```python
from build123d import *

# Parameters (mm, degrees)
F1_DEPTH = 10
F2_R     = 25.98667
F3_DEPTH = 20


with BuildPart() as f1:
    # F0 (on Front) → F1 (new body)
    with BuildSketch(Plane.XZ):
        Polygon((10.844505, -56.802116), (54.614328, -19.009441), (43.769823, 37.792675), (-10.844505, 56.802116), (-54.614328, 19.009441), (-43.769823, -37.792675), align=None)
    extrude(amount=F1_DEPTH)

    # F2 (on Front) → F3 (join)
    with BuildSketch(Plane.XZ):
        Circle(F2_R)
    extrude(amount=F3_DEPTH)


solid = f1.part
```
Design review of the part built by this model. Coordinates are the model's own, in mm. A direction names the side the tool comes from. Round coordinates to 2 decimals unless told otherwise and drop trailing zeros. Order: outer loops, then holes, each group sorted by start corner. A loop starts at its lowest first (then second) coordinate and runs counter-clockwise, first axis right, second up. Notation, with made-up numbers: (-12, 24.25) - (6, 24.25) arc R17 ccw to (6, 49.25) - close; hole circle Ø10 at (62.5, 60). An arc over 180 degrees is marked (long way). Return JSON: item names as keys, results as strings.
Q1. Consider section B-B on x = 0. Write out the cut boundary in (y, z).
Computed values:
{"outline": "(-20, -25.99) - (-10, -25.99) - (-10, -53.03) - (0, -53.03) - (0, 53.03) - (-10, 53.03) - (-10, 25.99) - (-20, 25.99) - close"}
Q2. Wall thickness on L1, parallel to Y at x = -6, z = 44.5; L2, parallel to X at y = -9, z = 34; L3, parallel to Z at x = 9, y = -19: over which ranges is each line inside the solid? List them lowest first. Write a range as [from, to].
Computed values:
{"L1": "y = [-10, 0]", "L2": "x = [-37.25, 44.49]", "L3": "z = [-24.38, 24.38]"}
Q3. Machinability: for faces 1 (the flat face through (24, -10, 13)), 2 (the flat face through (-16.845, -4.93, -47.164)), which of the approach directions +Z, -Z, +X, -X, +Y, -Y give a long, thin tool a straight path to every point of the face, cutting with its end or side? Answer none if there is none.
Computed values:
{"face 1": "-Y", "face 2": "-Z, -X, +Y, -Y"}
Q4. Consider section C-C on z = 0. Write out the cut boundary in (x, y).
Computed values:
{"outline": "(-50.99, -10) - (-25.99, -10) - (-25.99, -20) - (25.99, -20) - (25.99, -10) - (50.99, -10) - (50.99, 0) - (-50.99, 0) - close"}
Q5. For pin 1 Ø5 at (y, z) = (-12, -7) entering from +X; pin 2 Ø4 at (y, z) = (-10.5, -37.5) entering from +X; pin 3 Ø12 at (x, y) = (-1, -8) entering from +Z, all flat-tipped, find the tip position at first contact; note any pin that passes through.
Computed values:
{"pin 1": "stops at x = 52.61", "pin 2": "stops at x = 35.44", "pin 3": "stops at z = 55.46"}
Q6. Consider section D-D on x = -34. Write out the cut boundary in (y, z), plus the area to 3 significant figures.
Computed values:
{"outline": "(-10, -41.19) - (0, -41.19) - (0, 36.81) - (-10, 36.81) - close", "area": "780 mm2"}
Q7. Consider section A-A on y = -4. Write out the cut boundary in (x, z).
Computed values:
{"outline": "(-54.61, 19.01) - (-43.77, -37.79) - (10.84, -56.8) - (54.61, -19.01) - (43.77, 37.79) - (-10.84, 56.8) - close"}
